For this review, take the finished solid that the model builds, in its own axes (mm). Face numbers are marked on the shaded views. A direction names the side the tool comes from. Coordinates: 2 decimals unless noted, no trailing zeros. Loops run counter-clockwise (first coordinate to the right, second up) from the corner with the lowest first, then second, coordinate; pieces in that order, holes last. Notation, with made-up numbers: M 16.25,65 L 75.25,65 A27 ccw 75.25,84 Z; hole C 8.25,32.25 d6. An arc over 180 degrees is marked long. Use one line per item in the form item = value.
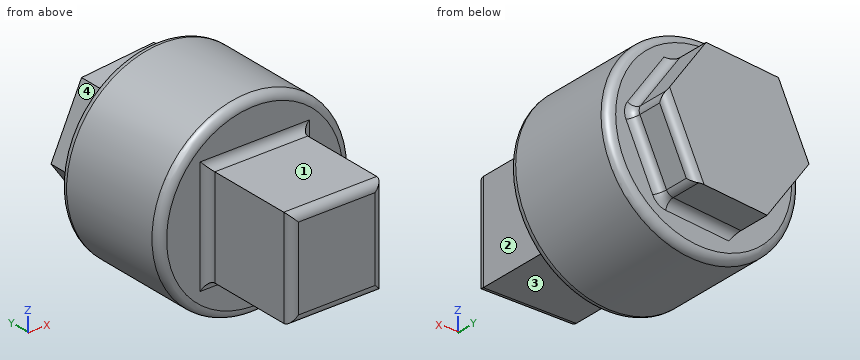
```python
from build123d import *

# Parameters (mm, degrees)
F0_R     = 60.3524841782
F1_DEPTH = 76.2
F3_W     = 58.3018623292
F3_H     = 61.5784339607
F4_DEPTH = 63.5
F7_DEPTH = 25.4
F8_F1_R  = 5.08
F8_F2_R  = 5.08
F9_R     = 5.08
F10_R    = 5.08


with BuildPart() as f1:
    # F0 (on Front) → F1 (new body)
    with BuildSketch(Plane.XZ):
        Circle(F0_R)
    extrude(amount=F1_DEPTH)

    # F3 (on face) → F4 (join)
    with BuildSketch(Plane.XZ.offset(76.2)):
        Rectangle(F3_W, F3_H)
    extrude(amount=F4_DEPTH)

    # F6 (on face) → F7 (join)
    with BuildSketch(Plane(origin=(0, 0, 0), x_dir=(-1, 0, 0), z_dir=(0, 1, 0))):
        Polygon((19.1640303054, -41.3700494554), (45.4095289369, -4.0884876443), (26.2454986315, 37.2815618111), (-19.1640303054, 41.3700494554), (-45.4095289369, 4.0884876443), (-26.2454986315, -37.2815618111), align=None)
    extrude(amount=F7_DEPTH)

    # F8: fillet of radius 5.08 on 4 edges, made by hand

    # F8_f1
    f8_f1_edges = [f1.edges().sort_by_distance(p)[0] for p in [
        (45.4095289369, 12.7, 4.0884876443),
        (26.2454986315, 12.7, -37.2815618111),
        (35.8275137842, 25.4, -16.5965370834),
    ]]
    fillet(f8_f1_edges, radius=F8_F1_R)

    # F8_f2
    f8_f2_edges = [f1.edges().sort_by_distance(p)[0] for p in [
        (35.8275137842, 0, -16.5965370834),
        (44.6268163137, 0, 4.0180154116),
        (25.7931115761, 0, -36.6389489119),
    ]]
    fillet(f8_f2_edges, radius=F8_F2_R)

    # F9
    f9_edges = [f1.edges().sort_by_distance(p)[0] for p in [
        (0, -139.7, -30.789217),
        (29.150931, -139.7, 0),
        (0, -139.7, 30.789217),
        (-29.150931, -139.7, 0),
        (-60.352484, -76.2, 0),
        (0, -76.2, -30.789217),
        (29.150931, -76.2, 0),
        (0, -76.2, 30.789217),
        (-29.150931, -76.2, 0),
    ]]
    fillet(f9_edges, radius=F9_R)

    # F10
    f10_edges = [f1.edges().sort_by_distance(p)[0] for p in [
        (-60.352484, 0, 0),
    ]]
    fillet(f10_edges, radius=F10_R)


solid = f1.part
```
1. Tool access review of the marked faces 1, 2, 3 and 4: name each direction out of +Z, -Z, +X, -X, +Y, -Y from which nothing blocks a thin tool from reaching the whole face with its end or side.
Computed values:
face_1 = +Z, +X, -X, -Y
face_2 = +Z, -Z, +X, -Y
face_3 = -Z, +X, -X, -Y
face_4 = +Z, -X, +Y
2. Consider section B-B on y = -110. Write out the cut boundary in (x, z), plus the area to 3 significant figures.
Computed values:
outline = M -29.15,-30.79 L 29.15,-30.79 L 29.15,30.79 L -29.15,30.79 Z
area = 3,590 mm2
3. Consider section A-A on y = -57. Write out the cut boundary in (x, z).
Computed values:
outline = C 0,0 d120.7
4. Wall thickness on line 1 along X through (y, z) = (-124, 24); line 2 along Y through (x, z) = (39, 38); line 3 along Z through (x, y) = (6, -130.5): over which ranges is each line inside the solid? List them lowest first. Write a range as from..to.
Computed values:
line_1 = -29.15..29.15
line_2 = -76.2..0
line_3 = -30.79..30.79
5. For pin 1 Ø6 at (y, z) = (-56, -20.5) entering from +X; pin 2 Ø6 at (x, z) = (-23.5, -41) entering from -Y; pin 3 Ø3 at (x, z) = (-36, 35) entering from +Y, all flat-tipped, find the tip position at first contact; note any pin that passes through.
Computed values:
pin_1 = 57.76
pin_2 = -76.2
pin_3 = 0
